For this review, use the dimensioned drawing (mm, ordinates from the lowest corner) and the shaded views. Coordinates: 2 decimals unless noted, no trailing zeros. Order: outer loops, then holes, each group sorted by start corner. A loop starts at its lowest first (then second) coordinate and runs counter-clockwise, first axis right, second up. Notation, with made-up numbers: M 1,32.5 L 35,32.5 A15 ccw 35,51.5 Z; hole C -33,51.25 d9. An arc over 180 degrees is marked long. Use CSV: the item, a comma, the result in double quotes.
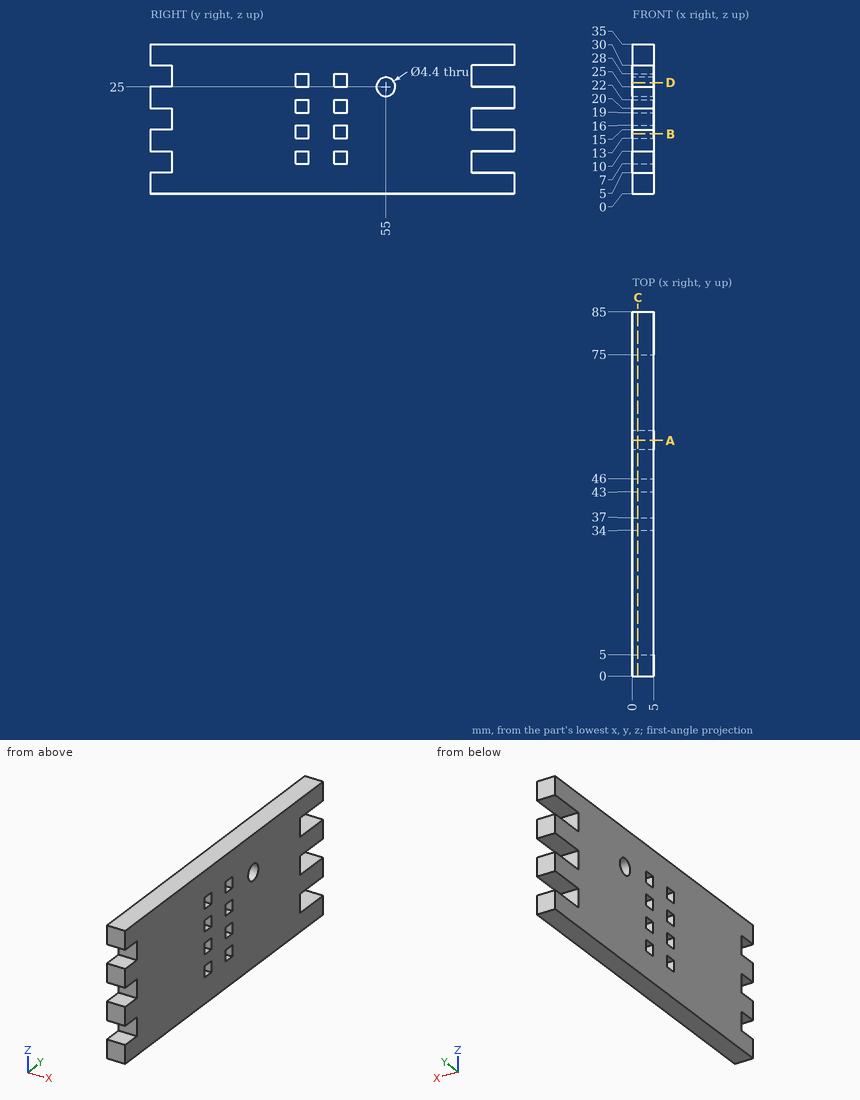
Item 1: Add section B-B on z = 14. State the section outline as (x, y) points.
Solutions:
outline,"M 0,0 L 5,0 L 5,34 L 0,34 Z; M 0,37 L 5,37 L 5,43 L 0,43 Z; M 0,46 L 5,46 L 5,85 L 0,85 Z"
Item 2: Add section A-A on y = 55. State the section outline as (x, z) points.
Solutions:
outline,"M 0,0 L 5,0 L 5,22.8 L 0,22.8 Z; M 0,27.2 L 5,27.2 L 5,35 L 0,35 Z"
Item 3: To check wall thickness, follow line 1 along Y through (x, z) = (1.8, 21.5); line 2 along Z through (x, y) = (1.9, 44.5); line 3 along Y through (x, z) = (0.65, 24.5). State the ranges of each line that lie inside material, in increasing order. Write a range as [from, to].
Solutions:
line 1,"[0, 34], [37, 43], [46, 85]"
line 2,"[0, 7], [10, 13], [16, 19], [22, 25], [28, 35]"
line 3,"[0, 52.86], [57.14, 85]"
Item 4: Add section C-C on x = 1.3. State how many separate pieces and enclosed holes the cut face has, and give its area (3 significant figures).
Solutions:
separate pieces,"1"
enclosed holes,"9"
area,"2,660 mm^2"
Item 5: Add section D-D on z = 26. State the section outline as (x, y) points.
Solutions:
outline,"M 0,5 L 5,5 L 5,34 L 0,34 Z; M 0,37 L 5,37 L 5,43 L 0,43 Z; M 0,46 L 5,46 L 5,53.04 L 0,53.04 Z; M 0,56.96 L 5,56.96 L 5,75 L 0,75 Z"
Item 6: Clearance check with a flat-ended pin moving along its axis: pin 1 Ø1.5 at (x, z) = (1.5, 18) entering from -Y. State where the tip first meets the part, or that it passes through.
Solutions:
pin 1,"y = 5"
